from build123d import *

# Parameters (mm, degrees)
SKETCH1_W           = 6
SKETCH1_H           = 4
SKETCH1_H_2         = 1
BOSS_EXTRUDE1_DEPTH = 5
SKETCH2_R           = 2.1
CUT_EXTRUDE1_DEPTH  = 6


with BuildPart() as part:
    # Sketch1 → Boss-Extrude1 (new body, symmetric)
    with BuildSketch(Plane.XY):
        Polygon((-5, 1.5), (-5, -1), (-3.5, -2.5), (-3, -2.5), (-3, 1.5), align=None)
        with Locations((0, -0.5)):
            Rectangle(SKETCH1_W, SKETCH1_H)
        with Locations((0, 2)):
            Rectangle(SKETCH1_W, SKETCH1_H_2)
        Polygon((3, 1.5), (3, -2.5), (3.5, -2.5), (5, -1), (5, 1.5), align=None)
    extrude(amount=BOSS_EXTRUDE1_DEPTH, both=True)

    # Sketch2 → Cut-Extrude1 (cut, through all)
    with BuildSketch(Plane(origin=(0, 2.5, 0), x_dir=(1, 0, 0), z_dir=(0, 1, 0))):
        Circle(SKETCH2_R)
    extrude(amount=-CUT_EXTRUDE1_DEPTH, mode=Mode.SUBTRACT)


solid = part.part
CAD build for the part. Positions are in the model's coordinates, mm. A direction names the side the tool comes from. Give positions to 0.01 mm unless a question says otherwise; leave off trailing zeros. Loops run counter-clockwise (first coordinate to the right, second up) from the corner with the lowest first, then second, coordinate; pieces in that order, holes last. Notation, with made-up numbers: M -18,-19 L -7,-19 A24 ccw -7,3 Z; hole C -16,-19.75 d11. An arc over 180 degrees is marked long. One line per question, with ' | ' between items. Start each with the question number.
1. Saw through at B-B on y = -2.05. Give the cut face in (x, z), plus the area to 3 significant figures.
2. Probe L1, parallel to Z at x = 0, y = 0.3; L2, parallel to Y at x = -3.25, z = -4. List the from-to ranges inside material, lowest first. Write a range as from..to.
3. 3-axis set-ups, long thin cutter, end or side, ignore diameter. For faces 1 (the face through (4, 1.5, 0)), 2 (the face through (-5, 0, 0)), 3 (the face through (-4, 1.5, 0)): which of +Z, -Z, +X, -X, +Y, -Y reach the whole face in a straight line?
4. Two-plate mould, pull along Z, no slides. Class faces 4 (the face through (2.003, 0.035, -0.631)), 5 (the face through (0, 0, -5)), 6 (the face through (-3, 2, 0)): pulls with the +Z half, pulls with the -Z half, needs draft (parallel to the pull), parting line crosses it, or undercut.
5. Saw through at D-D on z = -2.5. Give the cut face in (x, y), plus the area to 4 significant figures.
6. Flat gauge pins, fed straight in: pin 1 (6 mm diameter, centred on x = -2, z = 0, fed in from +Y); pin 2 (1.6 mm diameter, centred on x = -4, z = 0, fed in from +Y). Where does each tip first touch, or does it go through?
7. Saw through at A-A on x = 0. Give the cut face in (y, z).
8. Saw through at C-C on z = 0. Give the cut face in (x, y).
Result sheet:
1) outline: M -3.95,-5 L 3.95,-5 L 3.95,5 L -3.95,5 Z; hole C 0,0 d4.2 | area: 65.1 mm^2
2) L1: z = -5..-2.1, 2.1..5 | L2: y = -2.5..1.5
3) face 1: +Z, -Z, +X, +Y | face 2: +Z, -Z, -X, +Y, -Y | face 3: +Z, -Z, -X, +Y
4) face 4: undercut | face 5: pulls with the -Z half | face 6: needs draft
5) outline: M -5,-1 L -3.5,-2.5 L 3.5,-2.5 L 5,-1 L 5,1.5 L 3,1.5 L 3,2.5 L -3,2.5 L -3,1.5 L -5,1.5 Z | area: 43.75 mm^2
6) pin 1: stops at y = 2.5 | pin 2: stops at y = 1.5
7) outline: M -2.5,-5 L 2.5,-5 L 2.5,-2.1 L -2.5,-2.1 Z; M -2.5,2.1 L 2.5,2.1 L 2.5,5 L -2.5,5 Z
8) outline: M -5,-1 L -3.5,-2.5 L -2.1,-2.5 L -2.1,2.5 L -3,2.5 L -3,1.5 L -5,1.5 Z; M 2.1,-2.5 L 3.5,-2.5 L 5,-1 L 5,1.5 L 3,1.5 L 3,2.5 L 2.1,2.5 Z
